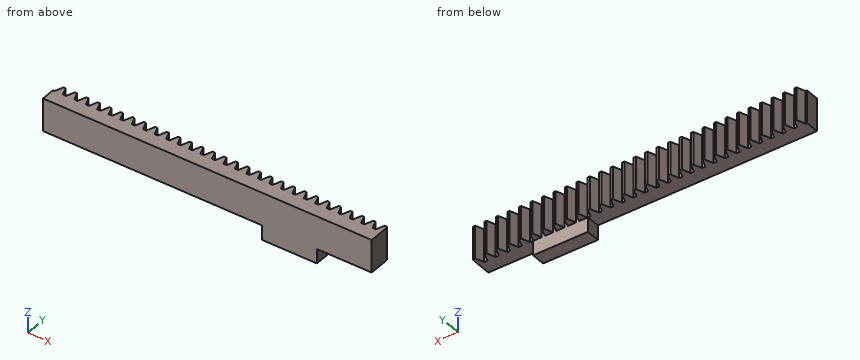
from build123d import *

# Parameters (mm, degrees)
BLANKSKE_W          = 90
BLANKSKE_H          = 6
BLANK_DEPTH         = 12
TOOTHCUTSIM_DEPTH   = 91.994505329
TEETHCUTS_COUNT     = 30
TEETHCUTS_PITCH     = 3.14159265
SKETCH3_W           = 91.493811728
SKETCH3_H           = 3
CUT_EXTRUDE3_DEPTH  = 10
SKETCH4_W           = 15
SKETCH4_H           = 3.75
BOSS_EXTRUDE1_DEPTH = 4


with BuildPart() as part:
    # BlankSke → Blank (new body)
    with BuildSketch(Plane.XY):
        with Locations((45, 3)):
            Rectangle(BLANKSKE_W, BLANKSKE_H)
    extrude(amount=-BLANK_DEPTH)

    # TooCutSkeSim → ToothCutSim (cut, through all)
    with BuildSketch(Plane.XY):
        Polygon((0.44443537, 3.75), (-0.44443537, 3.75), (-1.272613241, 6.0254), (1.272613241, 6.0254), align=None)
    toothcutsim = extrude(amount=-TOOTHCUTSIM_DEPTH, mode=Mode.SUBTRACT)

    # TeethCuts: ToothCutSim ×30
    with Locations(*[(i * TEETHCUTS_PITCH, 0, 0) for i in range(1, TEETHCUTS_COUNT)]):
        add(toothcutsim, mode=Mode.SUBTRACT)

    # Sketch3 → Cut-Extrude3 (cut)
    with BuildSketch(Plane(origin=(0, 0, 0), x_dir=(1, 0, 0), z_dir=(0, 1, 0))):
        with Locations((45.746905864, 10.5)):
            Rectangle(SKETCH3_W, SKETCH3_H)
    extrude(amount=CUT_EXTRUDE3_DEPTH, mode=Mode.SUBTRACT)

    # Sketch4 → Boss-Extrude1 (add)
    with BuildSketch(Plane(origin=(0, 0, -9), x_dir=(-1, 0, 0), z_dir=(0, 0, -1))):
        with Locations((-67.5, 1.875)):
            Rectangle(SKETCH4_W, SKETCH4_H)
    extrude(amount=BOSS_EXTRUDE1_DEPTH)


solid = part.part
Could you check a few things on this model? Use its own coordinates, in mm. Round coordinates to 2 decimals unless told otherwise and drop trailing zeros. Write each loop counter-clockwise with the first axis right and the second up, starting at its lowest first coordinate (ties: lowest second). Pieces come first, ordered by that corner, then holes. Notation, with made-up numbers: (-25.5, -0.75) -> (16.5, -0.75) arc R10 cw to (16.5, 3.25) -> close; hole circle Ø6 at (73.25, 34). An arc over 180 degrees is marked (long way). Use a Markdown table: item, result.
1. For pin 1 Ø1 at (x, y) = (29.5, 0.5) entering from -Z; pin 2 Ø1.9 at (y, z) = (1, -12) entering from +X; pin 3 Ø1.1 at (y, z) = (1, -10.5) entering from -X, each with a flat end and sliding along its axis, tell me the tip position at first contact or that it passes through.
Answer key:
| item | result |
|---|---|
| pin 1 | stops at z = -9 |
| pin 2 | stops at x = 75 |
| pin 3 | stops at x = 60 |
2. Please list where these lines run through material, in increasing order: probe 1 along Y at (x, z) = (69, -12); probe 2 along Z at (x, y) = (11.5, 5); probe 3 along X at (y, z) = (1, -10.5).
Answer key:
| item | result |
|---|---|
| probe 1 | y = 0 to 3.75 |
| probe 2 | z = -9 to 0 |
| probe 3 | x = 60 to 75 |
3. If we section it at A-A (y = 3): List the corners of the cut face in (x, z) for me, then the cut area to 3 significant figures.
Answer key:
| item | result |
|---|---|
| outline | (0, -9) -> (60, -9) -> (60, -13) -> (75, -13) -> (75, -9) -> (90, -9) -> (90, 0) -> (0, 0) -> close |
| area | 870 mm^2 |
4. If we section it at B-B (z = -10): List the corners of the cut face in (x, y) for me.
Answer key:
| item | result |
|---|---|
| outline | (60, 0) -> (75, 0) -> (75, 3.75) -> (60, 3.75) -> close |
